Part model, mm, in its own coordinate system. Face numbers are marked on the shaded views. Give positions to 0.01 mm unless a question says otherwise; leave off trailing zeros. Write each loop counter-clockwise with the first axis right and the second up, starting at its lowest first coordinate (ties: lowest second). Pieces come first, ordered by that corner, then holes. Notation, with made-up numbers: M 54.5,77 L 90.5,77 A8 ccw 90.5,82 Z; hole C 4,63.25 d2. An arc over 180 degrees is marked long. Answer as CSV lines item,"result". Start each with the question number.
Item 1: Two-plate mould, pull along Y, no slides. Class the marked faces 1, 2 and 3: +Y half, -Y half, draft (parallel to the pull), parting line (faces both ways), or undercut.
Item 2: Band-saw the part on C-C, the plane z = 7.5. List the corners of the cut face in (x, y), then the cut area to 3 significant figures.
Item 3: Wall check: L1, parallel to X at y = -0.5, z = 26; L2, parallel to Z at x = 1.5, y = -10.5; L3, parallel to Z at x = 0, y = 37. Give the ranges that are in metal, low to high. Write a range as from..to.
Item 4: Band-saw the part on B-B, the plane z = 38. List the corners of the cut face in (x, y), then the cut area to 3 significant figures.
Item 5: Band-saw the part on D-D, the plane x = -1.5. Count the separate pieces of the cut face and the enclosed holes in it, then the cut area to 3 significant figures.
Item 6: Band-saw the part on A-A, the plane y = 0. List the corners of the cut face in (x, z).
Item 7: Pin check, flat tips, straight feed: pin 1 (1 mm diameter, centred on x = 30, z = 23, fed in from -Y); pin 2 (3 mm diameter, centred on y = -17.5, z = 42, fed in from +X); pin 3 (3 mm diameter, centred on x = 2, z = 41.5, fed in from +Y); pin 4 (5 mm diameter, centred on x = 0, z = 38, fed in from +Y). Stop position of each tip, or through.
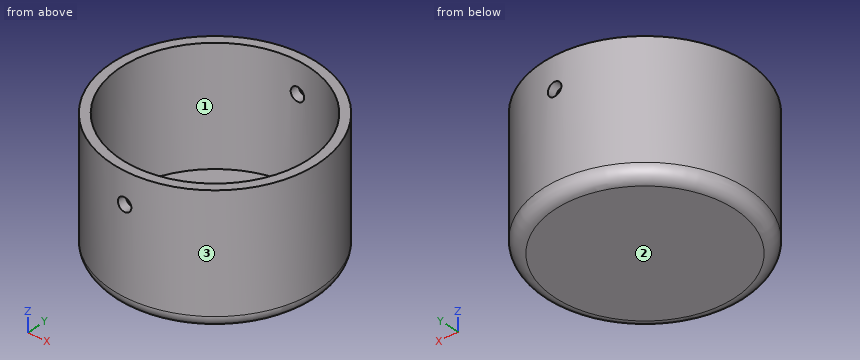
from build123d import *

# Parameters (mm, degrees)
F0_R     = 40
F0_R_2   = 36.5
F1_DEPTH = 5
F2_DEPTH = 50
F3_R     = 2.65
F4_DEPTH = 75
F5_R     = 5


with BuildPart() as f1:
    # F0 (on Top) → F1 (new body)
    with BuildSketch(Plane.XY):
        Circle(F0_R)
        Circle(F0_R_2, mode=Mode.SUBTRACT)
        Circle(F0_R_2)
    extrude(amount=F1_DEPTH)

    # F0 (on Top) → F2 (join)
    with BuildSketch(Plane.XY):
        Circle(F0_R)
        Circle(F0_R_2, mode=Mode.SUBTRACT)
    extrude(amount=F2_DEPTH)

    # F3 (on Front) → F4 (cut, symmetric)
    with BuildSketch(Plane.XZ):
        with Locations((0, 38)):
            Circle(F3_R)
    extrude(amount=F4_DEPTH, both=True, mode=Mode.SUBTRACT)

    # F5
    f5_edges = [f1.edges().sort_by_distance(p)[0] for p in [
        (-40, 0, 0),
    ]]
    fillet(f5_edges, radius=F5_R)


solid = f1.part
Output:
1,face 1,"undercut"
1,face 2,"draft"
1,face 3,"parting line"
2,outline,"C 0,0 d80; hole C 0,0 d73"
2,area,"841 mm²"
3,L1,"-40..-36.5, 36.5..40"
3,L2,"0..5"
3,L3,"0.42..35.35, 40.65..50"
4,outline,"M -2.65,-39.91 L -2.65,-36.4 A36.5 cw -2.65,36.4 L -2.65,39.91 A40 ccw Z; M 2.65,-39.91 A40 ccw 2.65,39.91 L 2.65,36.4 A36.5 cw 2.65,-36.4 Z"
4,area,"804 mm²"
5,separate pieces,"3"
5,enclosed holes,"0"
5,area,"674 mm²"
6,outline,"M -40,5 A5 ccw -35,0 L 35,0 A5 ccw 40,5 L 40,50 L 36.5,50 L 36.5,5 L -36.5,5 L -36.5,50 L -40,50 Z"
7,pin 1,"y = -27.01"
7,pin 2,"x = 36.66"
7,pin 3,"y = 40"
7,pin 4,"through"
